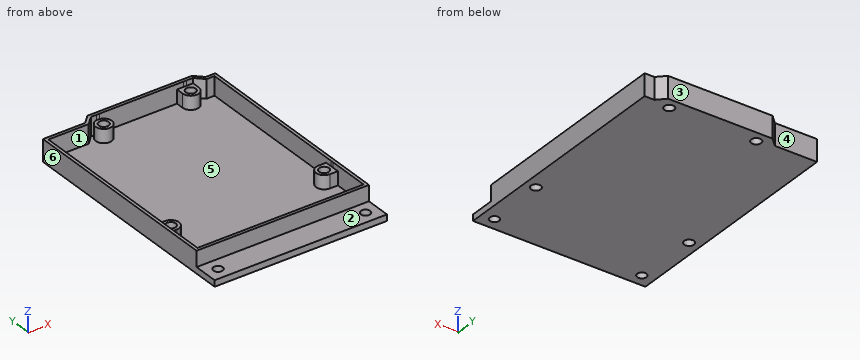
Autodesk Inventor part; units mm, degrees
ref_plane "YZ Plane" through (0, 0, 0) normal (1, 0, 0) x (0, 1, 0)
ref_plane "XZ Plane" through (0, 0, 0) normal (0, 1, 0) x (-1, 0, 0)
ref_plane "XY Plane" through (0, 0, 0) normal (0, 0, 1) x (1, 0, 0)
sketch "Esquisse8" plane through (0, 0, 0) normal (0, 0, 1) x (1, 0, 0)
  line L0 (0, 66.04) -> (0, 0)
  line L1 (0, 0) -> (0, 66.04)
  line L2 (12.954, 66.04) -> (0, 66.04)
  line L3 (0, 66.04) -> (12.954, 66.04)
  line L4 (48.26, 68.58) -> (15.494, 68.58)
  line L5 (12.954, 66.04) -> (15.494, 68.58)
  line L6 (50.8, 66.04) -> (48.26, 68.58)
  line L7 (15.494, 68.58) -> (48.26, 68.58)
  line L8 (48.26, 68.58) -> (50.8, 66.04)
  line L9 (53.34, 0) -> (53.34, 66.04)
  line L10 (50.8, 66.04) -> (53.34, 66.04)
  line L11 (53.34, 66.04) -> (53.34, 0)
  line L12 (53.34, 0) -> (0, 0)
  circle A0 centre (2.54, 15.24) radius 1.5875
  circle A1 centre (2.54, 15.24) radius 1.5875
  circle A2 centre (50.8, 13.97) radius 1.5875
  circle A3 centre (50.8, 13.97) radius 1.5875
  circle A4 centre (45.72, 66.04) radius 1.5875
  circle A5 centre (45.72, 66.04) radius 1.5875
  circle A6 centre (17.78, 66.04) radius 1.5875
  circle A7 centre (17.78, 66.04) radius 1.5875
  line L13 (15.0798, 69.58) -> (48.6742, 69.58)
  line L14 (51.2142, 67.04) -> (48.6742, 69.58)
  line L15 (51.2142, 67.04) -> (54.34, 67.04)
  line L16 (54.34, -1) -> (54.34, 67.04)
  line L17 (54.34, -1) -> (-1, -1)
  line L18 (-1, -1) -> (-1, 67.04)
  line L19 (-1, 67.04) -> (12.5398, 67.04)
  line L20 (12.5398, 67.04) -> (15.0798, 69.58)
  dimension "d59" = 1
  dimension "d60" = 1
  dimension "d61" = 1
  dimension "d62" = 1
  dimension "d63" = 1
  dimension "d64" = 1
  dimension "d65" = 1
extrude "Extrusion5" add sketch "Esquisse8" along normal blind 7 contours L2 L5 L4 L6 L10 L9 L12 L0 | L13 L14 L15 L16 L17 L18 L19 L20
shell "Coque1" thickness 1 removed faces 1 at (23.8943, 31.957, 7)
sketch "Esquisse10" plane through (0, 0, 1) normal (0, 0, 1) x (1, 0, 0)
  arc A0 (0, 14.7465) -> (0, 15.7335) centre (2.54, 15.24) ccw
  line L0 (2.54, 17.8275) -> (0, 17.8275)
  arc A1 (53.34, 14.4635) -> (53.34, 13.4765) centre (50.8, 13.97) ccw
  line L1 (50.8, 16.5575) -> (53.34, 16.5575)
  line L2 (50.8, 11.3825) -> (53.34, 11.3825)
  arc A2 (45.2265, 68.58) -> (46.2135, 68.58) centre (45.72, 66.04) ccw
  line L3 (43.1325, 66.04) -> (43.1325, 68.58)
  line L4 (48.3075, 66.04) -> (48.3075, 68.58)
  circle A3 centre (2.54, 15.24) radius 2.5875
  line L5 (0, 17.8275) -> (0, 12.6525)
  line L6 (0, 15.7335) -> (0, 66.04)
  line L7 (53.34, 16.5575) -> (53.34, 11.3825)
  line L8 (53.34, 66.04) -> (53.34, 14.4635)
  line L9 (43.1325, 68.58) -> (48.3075, 68.58)
  line L10 (18.2735, 68.58) -> (45.2265, 68.58)
  circle A4 centre (45.72, 66.04) radius 1.5875
  circle A5 centre (45.72, 66.04) radius 2.5875
  circle A6 centre (50.8, 13.97) radius 1.5875
  circle A7 centre (50.8, 13.97) radius 2.5875
  line L11 (2.54, 12.6525) -> (0, 12.6525)
  line L12 (0, 0) -> (0, 14.7465)
extrude "Extrusion6" add sketch "Esquisse10" along normal blind 4.35 contours L5 L0 A0 | L7 A1 | A1 L1 L7 | L7 L2 A1 | L9 A2 | A2 L3 L9 | L9 L4 A2
sketch "Esquisse11" plane through (0, 0, 7) normal (0, 0, 1) x (1, 0, 0)
  arc A0 (0, 14.7465) -> (2.54, 17.8275) centre (2.54, 15.24) ccw
  line L0 (2.54, 12.6525) -> (0, 12.6525)
  line L1 (0, 0) -> (0, 14.7465)
  line L2 (0, 12.6525) -> (0, 14.7465)
  circle A1 centre (2.54, 15.24) radius 2.5875
extrude "Extrusion7" add sketch "Esquisse11" against normal blind 6 contours A0 L0 L1
sketch "Esquisse12" plane through (0, 0, 0) normal (0, 0, -1) x (-1, 0, 0)
  line L0 (-54.34, -1) -> (1, -1)
  line L1 (1, -1) -> (1, -9)
  line L2 (1, -9) -> (-54.34, -9)
  line L3 (-54.34, -9) -> (-54.34, -1)
  point P0 (0, 0)
  dimension "d80" = 8
extrude "Extrusion8" add sketch "Esquisse12" against normal blind 2
sketch "Esquisse13" plane through (0, 0, 2) normal (0, 0, 1) x (1, 0, 0)
  line L0 (-1, -9) -> (54.34, -9)
  line L1 (-1, -9) -> (3, -9)
  line L2 (3, -9) -> (3, -1.5792)
  line L3 (-1, -9) -> (-1, 67.04)
  line L4 (-1, -9) -> (-1, -5)
  line L5 (-1, -5) -> (3, -5)
  line L6 (26.67, -9) -> (26.67, -6.1659)
  point P0 (0, 0)
  point P1 (50.34, -5)
  dimension "d83" = 4
  dimension "d84" = 4
hole "Perçage2" at (3, -5, 2) at (50.34, -5, 2) direction (0, 0, -1) diameter 3 end through all
sketch "Esquisse14" plane through (0, 0, 7) normal (0, 0, 1) x (1, 0, 0)
  line L0 (0, 0) -> (0, 12.6525)
  line L1 (0, 15.7335) -> (0, 17.8275)
  line L2 (0, 12.6525) -> (0, 15.7335)
  arc A0 (2.54, 12.6525) -> (0, 15.7335) centre (2.54, 15.24) ccw
  line L3 (0, 12.6525) -> (2.54, 12.6525)
  arc A1 (2.54, 12.6525) -> (0, 15.7335) centre (2.54, 15.24) ccw
  circle A2 centre (2.54, 15.24) radius 1.5875
  circle A3 centre (50.8, 13.97) radius 1.5875
  circle A4 centre (50.8, 13.97) radius 1.5875
  arc A5 (53.34, 14.4635) -> (53.34, 13.4765) centre (50.8, 13.97) ccw
  line L4 (53.34, 66.04) -> (53.34, 14.4635)
  line L5 (53.34, 14.4635) -> (53.34, 13.4765)
  arc A6 (48.3075, 66.04) -> (46.2135, 68.58) centre (45.72, 66.04) ccw
  line L6 (45.2073, 68.58) -> (46.2135, 68.58)
  circle A7 centre (45.72, 66.04) radius 1.5875
  circle A8 centre (45.72, 66.04) radius 1.5875
  arc A9 (45.2265, 68.58) -> (46.2135, 68.58) centre (45.72, 66.04) ccw
  circle A10 centre (17.78, 66.04) radius 1.5875
  circle A11 centre (17.78, 66.04) radius 1.5875
  arc A12 (17.2865, 68.58) -> (18.2735, 68.58) centre (17.78, 66.04) ccw
  arc A13 (17.2865, 68.58) -> (18.2735, 68.58) centre (17.78, 66.04) ccw
  line L7 (17.2865, 68.58) -> (18.2735, 68.58)
extrude "Extrusion9" cut sketch "Esquisse14" against normal blind 1.65 contours L2 A0 L3 | L5 A5
sketch "Esquisse15" plane through (0, 0, 7) normal (0, 0, 1) x (1, 0, 0)
  circle A0 centre (17.78, 66.04) radius 1.5875
  circle A1 centre (17.78, 66.04) radius 1.5875
  arc A2 (17.2865, 68.58) -> (18.2735, 68.58) centre (17.78, 66.04) ccw
  line L0 (15.494, 68.58) -> (17.2865, 68.58)
  line L1 (17.2865, 68.58) -> (18.2735, 68.58)
  circle A3 centre (45.72, 66.04) radius 1.5875
  circle A4 centre (45.72, 66.04) radius 1.5875
  arc A5 (45.2265, 68.58) -> (46.2135, 68.58) centre (45.72, 66.04) ccw
  line L2 (18.2735, 68.58) -> (45.2265, 68.58)
  arc A6 (45.2265, 68.58) -> (46.2135, 68.58) centre (45.72, 66.04) ccw
  line L3 (45.2265, 68.58) -> (46.2135, 68.58)
  point P0 (0, 0)
extrude "Extrusion10" cut sketch "Esquisse15" against normal blind 1.65
properties part number "Arduino+Support"
Design review of the part built by this model. Coordinates are the model's own, in mm. Face numbers are marked on the shaded views. A direction names the side the tool comes from. Coordinates: 2 decimals unless noted, no trailing zeros. Loops run counter-clockwise (first coordinate to the right, second up) from the corner with the lowest first, then second, coordinate; pieces in that order, holes last. Notation, with made-up numbers: (62, 2) -> (116, 2) arc R18 cw to (116, 26) -> close; hole circle Ø11 at (33, 86.5). An arc over 180 degrees is marked (long way). Answer as a JSON object with one key per item and string values.
Q1. Take a section at D-D on x = 9.5. Give the boundary of the cut face in (y, z).
Answer block:
{"outline": "(-9, 0) -> (67.04, 0) -> (67.04, 7) -> (66.04, 7) -> (66.04, 1) -> (0, 1) -> (0, 7) -> (-1, 7) -> (-1, 2) -> (-9, 2) -> close"}
Q2. Clearance check with flat-ended pins moving along their axes: pin 1 Ø1 at (x, y) = (6.5, 4.5) entering from +Z; pin 2 Ø4 at (x, y) = (50.8, 13.97) entering from +Z; pin 3 Ø0.5 at (x, z) = (45.5, 6) entering from -Y. State where each tip first meets the part, or that it passes through.
Answer block:
{"pin 1": "stops at z = 1", "pin 2": "stops at z = 5.35", "pin 3": "stops at y = -1"}
Q3. Tool access review of the marked faces 1, 2 and 3: name each direction out of +Z, -Z, +X, -X, +Y, -Y from which nothing blocks a thin tool from reaching the whole face with its end or side.
Answer block:
{"face 1": "+Z", "face 2": "+Z, +X, -X, -Y", "face 3": "+Z, -Z, +X, -X, +Y"}
Q4. To check wall thickness, follow L1, parallel to X at y = -5, z = 0.95; L2, parallel to Y at x = 45.72, z = 2.5; L3, parallel to X at y = 46.5, z = 2. State the ranges of each line that lie inside material, in increasing order.
Answer block:
{"L1": "x = -1 to 1.5, 4.5 to 48.84, 51.84 to 54.34", "L2": "y = -1 to 0, 63.45 to 64.45, 67.63 to 69.58", "L3": "x = -1 to 0, 53.34 to 54.34"}
Q5. Take a section at C-C on z = 3. Give the number of separate pieces and of enclosed holes in the cut face, plus the area to 3 significant figures.
Answer block:
{"separate pieces": "1", "enclosed holes": "5", "area": "305 mm^2"}
Q6. Take a section at B-B on x = 39.5. Give the boundary of the cut face in (y, z), plus the area to 3 significant figures.
Answer block:
{"outline": "(-9, 0) -> (69.58, 0) -> (69.58, 7) -> (68.58, 7) -> (68.58, 1) -> (0, 1) -> (0, 7) -> (-1, 7) -> (-1, 2) -> (-9, 2) -> close", "area": "98.6 mm^2"}
Q7. The part is to be moulded in two halves that separate along X. For the marked faces 4, 5 and 6, say which applies: +X half, -X half, draft (parallel to the pull), parting line (faces both ways), or undercut.
Answer block:
{"face 4": "draft", "face 5": "undercut", "face 6": "-X half"}
Q8. Take a section at A-A on y = 7. Give the boundary of the cut face in (x, z), plus the area to 3 significant figures.
Answer block:
{"outline": "(-1, 0) -> (54.34, 0) -> (54.34, 7) -> (53.34, 7) -> (53.34, 1) -> (0, 1) -> (0, 7) -> (-1, 7) -> close", "area": "67.3 mm^2"}
